Build history of the part. All positions in model axes, mm. Face numbers are marked on the shaded views. A direction names the side the tool comes from. Coordinates: 2 decimals unless noted, no trailing zeros. Write each loop counter-clockwise with the first axis right and the second up, starting at its lowest first coordinate (ties: lowest second). Pieces come first, ordered by that corner, then holes.
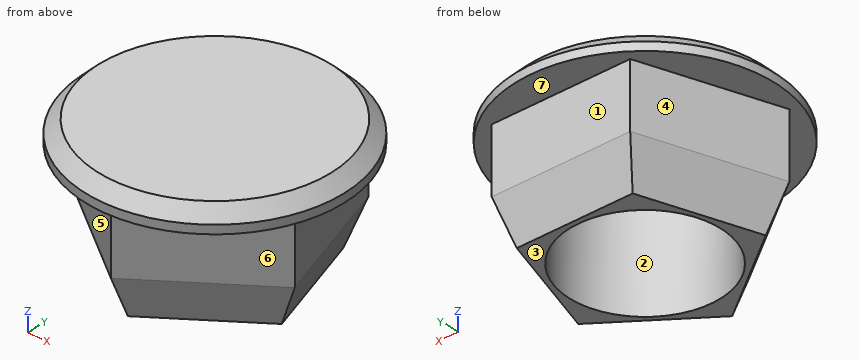
from build123d import *

# Parameters (mm, degrees)
F0_R     = 6
F1_DEPTH = 1
F2_SIZE  = 0.6
F3_R     = 3.5
F4_DEPTH = 5
F5_SIZE2 = 0.72794
F5_SIZE  = 2


with BuildPart() as f1:
    # F0 (on Top) → F1 (new body)
    with BuildSketch(Plane.XY):
        Circle(F0_R)
    extrude(amount=F1_DEPTH)

    # F2
    f2_edges = [f1.edges().sort_by_distance(p)[0] for p in [
        (-6, 0, 1),
    ]]
    chamfer(f2_edges, length=F2_SIZE)

    # F3 (on face) → F4 (join)
    with BuildSketch(Plane(origin=(0, 0, 0), x_dir=(1, 0, 0), z_dir=(0, 0, -1))):
        Polygon((5.230811, 1.699593), (0, 5.5), (-5.230811, 1.699593), (-3.232819, -4.449593), (3.232819, -4.449593), align=None)
        Circle(F3_R, mode=Mode.SUBTRACT)
    extrude(amount=F4_DEPTH)

    # F5
    f5_edges = [f1.edges().sort_by_distance(p)[0] for p in [
        (-2.615405, -3.599797, -5),
        (-4.231815, 1.375, -5),
        (0, 4.449593, -5),
        (4.231815, 1.375, -5),
        (2.615405, -3.599797, -5),
    ]]
    chamfer(f5_edges, length=F5_SIZE, length2=F5_SIZE2)


solid = f1.part
(1) Probe L1, parallel to Z at x = 1.25, y = 0; L2, parallel to Y at x = -0.75, z = -4.7; L3, parallel to Y at x = 3, z = -1.2. List the from-to ranges inside material, lowest first.
(2) Slice it at B-B, the plane y = 0. List the corners of the cut face in (x, z).
(3) Slice it at A-A, the plane z = -0.7. List the corners of the cut face in (x, y).
(4) Slice it at C-C, the plane z = -3.25. List the corners of the cut face in (x, y), and give its area (3 significant figures).
(5) Flat gauge pins, fed straight in: P1, Ø2, axis at x = 0, y = -1.5, coming from the -Z side; P2, Ø2, axis at y = 2, z = -3.5, coming from the -X side; P3, Ø1, axis at x = -3.5, z = -1, coming from the -Y side. Where does each tip first touch, or does it go through?
(6) Two-plate mould, pull along Y, no slides. Class the marked faces 1, 2 and 3: pulls with the +Y half, pulls with the -Y half, needs draft (parallel to the pull), parting line crosses it, or undercut.
(7) 3-axis set-ups, long thin cutter, end or side, ignore diameter. For the marked faces 4, 5, 6 and 7: which of +Z, -Z, +X, -X, +Y, -Y reach the whole face in a straight line?
Results:
1. L1: z = 0 to 1
1. L2: y = -4.19 to -3.42, 3.42 to 3.83
1. L3: y = -3.32 to -1.8, 1.8 to 4.45
2. outline: (-6, 0) - (-4.68, 0) - (-4.68, -3) - (-3.91, -5) - (-3.5, -5) - (-3.5, 0) - (3.5, 0) - (3.5, -5) - (3.91, -5) - (4.68, -3) - (4.68, 0) - (6, 0) - (6, 0.4) - (5.4, 1) - (-5.4, 1) - (-6, 0.4) - close
3. outline: (-5.23, -1.7) - (0, -5.5) - (5.23, -1.7) - (3.23, 4.45) - (-3.23, 4.45) - close; hole circle Ø7 at (0, 0)
4. outline: (-5.12, -1.66) - (0, -5.39) - (5.12, -1.66) - (3.17, 4.36) - (-3.17, 4.36) - close; hole circle Ø7 at (0, 0)
4. area: 30.5 mm2
5. P1: stops at z = 0
5. P2: stops at x = -4.31
5. P3: stops at y = -3.32
6. face 1: pulls with the +Y half
6. face 2: undercut
6. face 3: needs draft
7. face 4: -Z, -X, +Y
7. face 5: -Z, -X, -Y
7. face 6: -Z, +X, -Y
7. face 7: -Z
